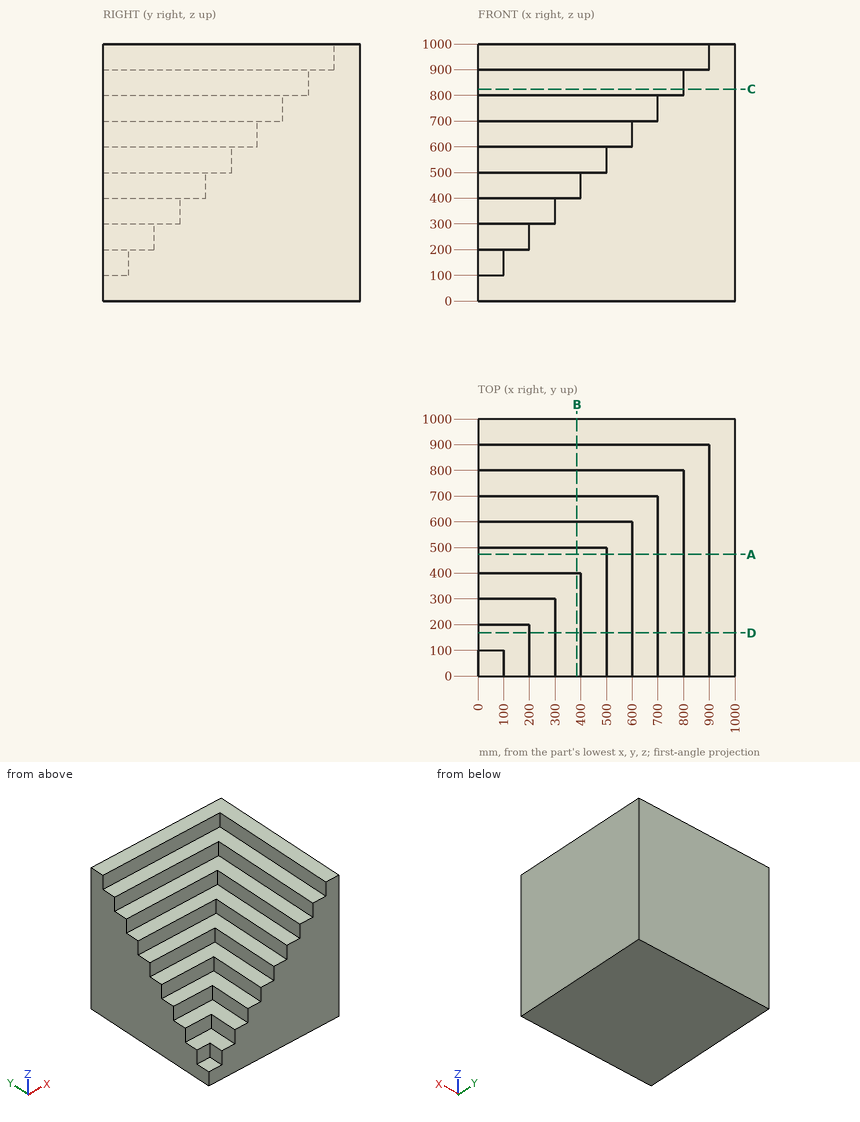
Check sheet for the drawn part. Datum: minimum x, y, z corner. Units: mm. Round coordinates to 2 decimals unless told otherwise and drop trailing zeros. Loops run counter-clockwise (first coordinate to the right, second up) from the corner with the lowest first, then second, coordinate; pieces in that order, holes last. Notation, with made-up numbers: (11, 11) -> (35, 11) arc R15 cw to (35, 23) -> close; hole circle Ø4 at (-10, 23.5). An arc over 180 degrees is marked (long way). Put each result on its own line as item: value. Start each with the question number.
1. Section check D-D (y = 167.5). Enter the section's corners in (x, z).
2. Scan lines: probe 1 along X at (y, z) = (775, 836); probe 2 along Z at (x, y) = (566, 773.5); probe 3 along Z at (x, y) = (214, 644). Record each from-to range of solid material in increasing order.
3. Section check A-A (y = 473.5). Enter the section's corners in (x, z), plus the area to 3 significant figures.
4. Gauge pin test, flat ends, axial feed: pin 1 (4 mm diameter, centred on y = 735, z = 510.5, fed in from -X); pin 2 (1.5 mm diameter, centred on y = 162.5, z = 484, fed in from -X); pin 3 (6 mm diameter, centred on x = 298.5, y = 401.5, fed in from +Z); pin 4 (8 mm diameter, centred on y = 115.5, z = 841.5, fed in from -X). Record the tip position at first contact, or that the pin passes through.
5. Section check B-B (x = 385). Enter the section's corners in (y, z), plus the area to 3 significant figures.
6. Section check C-C (z = 824.5). Enter the section's corners in (x, y).
Findings:
1. outline: (0, 0) -> (1000, 0) -> (1000, 1000) -> (900, 1000) -> (900, 900) -> (800, 900) -> (800, 800) -> (700, 800) -> (700, 700) -> (600, 700) -> (600, 600) -> (500, 600) -> (500, 500) -> (400, 500) -> (400, 400) -> (300, 400) -> (300, 300) -> (200, 300) -> (200, 200) -> (0, 200) -> close
2. probe 1: x = 800 to 1000
2. probe 2: z = 0 to 800
2. probe 3: z = 0 to 700
3. outline: (0, 0) -> (1000, 0) -> (1000, 1000) -> (900, 1000) -> (900, 900) -> (800, 900) -> (800, 800) -> (700, 800) -> (700, 700) -> (600, 700) -> (600, 600) -> (500, 600) -> (500, 500) -> (0, 500) -> close
3. area: 650,000 mm^2
4. pin 1: stops at x = 0
4. pin 2: stops at x = 400
4. pin 3: stops at z = 500
4. pin 4: stops at x = 800
5. outline: (0, 0) -> (1000, 0) -> (1000, 1000) -> (900, 1000) -> (900, 900) -> (800, 900) -> (800, 800) -> (700, 800) -> (700, 700) -> (600, 700) -> (600, 600) -> (500, 600) -> (500, 500) -> (400, 500) -> (400, 400) -> (0, 400) -> close
5. area: 610,000 mm^2
6. outline: (0, 800) -> (800, 800) -> (800, 0) -> (1000, 0) -> (1000, 1000) -> (0, 1000) -> close
